For this review, use the dimensioned drawing (mm, ordinates from the lowest corner) and the shaded views. A direction names the side the tool comes from. Coordinates: 2 decimals unless noted, no trailing zeros. Loops run counter-clockwise (first coordinate to the right, second up) from the corner with the lowest first, then second, coordinate; pieces in that order, holes last. Notation, with made-up numbers: (-10.5, -35.5) -> (31.5, -35.5) arc R22 cw to (31.5, -25.5) -> close; hole circle Ø11 at (-30.75, 56.25). An arc over 180 degrees is marked (long way). Answer as a JSON object with one key per item and string values.
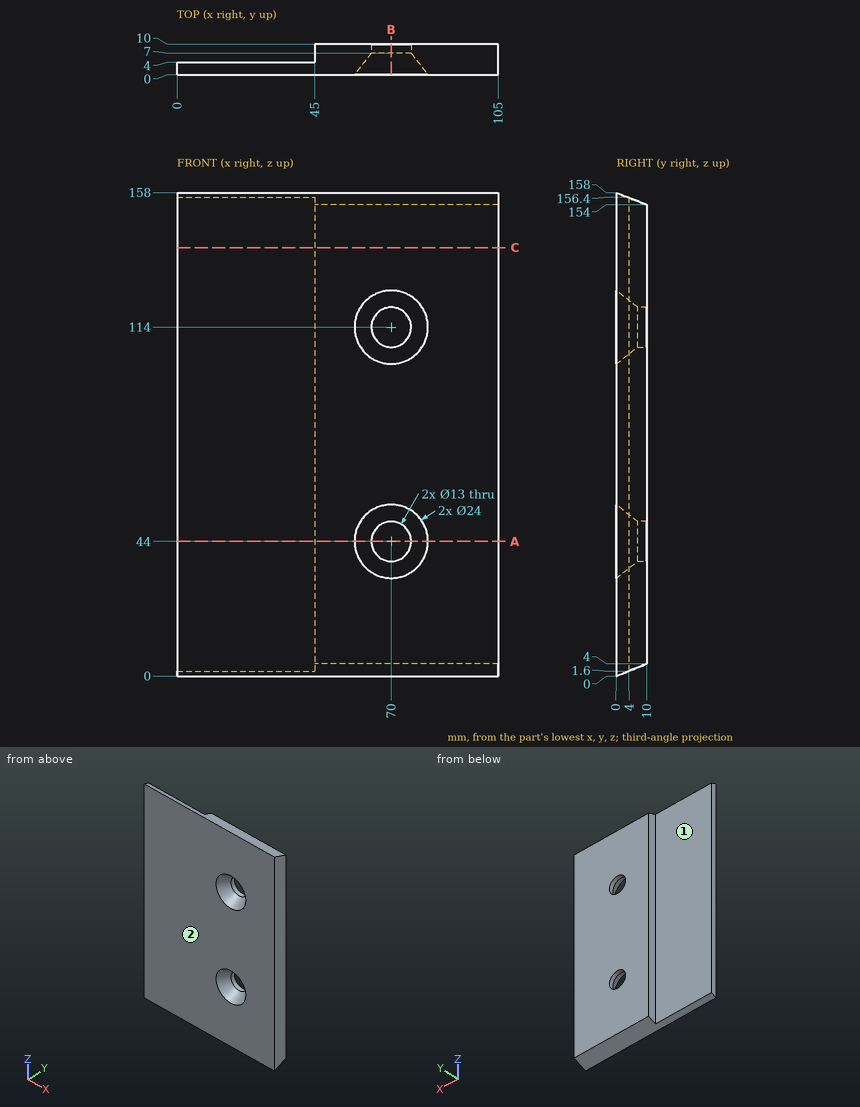
1) Wall thickness on probe 1 along X at (y, z) = (8.55, 44); probe 2 along Y at (x, z) = (19.5, 73); probe 3 along X at (y, z) = (1.5, 121): over which ranges is each line inside the solid? List them lowest first.
Completed:
{"probe 1": "45 to 63.5, 76.5 to 105", "probe 2": "0 to 4", "probe 3": "0 to 61.75, 78.25 to 105"}
2) Clearance check with flat-ended pins moving along their axes: pin 1 Ø3 at (x, y) = (16, 2) entering from +Z; pin 2 Ø2 at (x, y) = (76, 4) entering from -Z; pin 3 Ø3 at (y, z) = (7, 110.5) entering from -X. State where each tip first meets the part, or that it passes through.
Completed:
{"pin 1": "z = 157.8", "pin 2": "z = 1.2", "pin 3": "x = 45"}
3) Add section A-A, the plane z = 44. Give the boundary of the cut face in (x, y).
Completed:
{"outline": "(0, 0) -> (58, 0) -> (63.5, 7) -> (63.5, 10) -> (45, 10) -> (45, 4) -> (0, 4) -> close; (76.5, 7) -> (82, 0) -> (105, 0) -> (105, 10) -> (76.5, 10) -> close"}
4) Add section B-B, the plane x = 70. Give the boundary of the cut face in (y, z), and give its area (3 significant figures).
Completed:
{"outline": "(0, 0) -> (10, 4) -> (10, 37.5) -> (7, 37.5) -> (0, 32) -> close; (0, 56) -> (7, 50.5) -> (10, 50.5) -> (10, 107.5) -> (7, 107.5) -> (0, 102) -> close; (0, 126) -> (7, 120.5) -> (10, 120.5) -> (10, 154) -> (0, 158) -> close", "area": "1,200 mm²"}
5) Add section C-C, the plane z = 140. Give the boundary of the cut face in (x, y), and give its area (3 significant figures).
Completed:
{"outline": "(0, 0) -> (105, 0) -> (105, 10) -> (45, 10) -> (45, 4) -> (0, 4) -> close", "area": "780 mm²"}
6) For the marked faces 1 and 2, list the 3-axis set-ups (+Z, -Z, +X, -X, +Y, -Y) from which the entire face can be reached by the end or side of a thin tool; tool diameter is ignored.
Completed:
{"face 1": "+Z, -Z, -X, +Y", "face 2": "+Z, -Z, +X, -X, -Y"}
